```python
from build123d import *

# Parameters (mm, degrees)
BOSS_EXTRUDE2_DEPTH = 15
SKETCH3_W           = 40
SKETCH3_H           = 15
BOSS_EXTRUDE3_DEPTH = 10
BOSS_EXTRUDE4_START = -50
SKETCH4_R           = 5
BOSS_EXTRUDE4_DEPTH = 60
SKETCH5_W           = 20
SKETCH5_H           = 15
BOSS_EXTRUDE5_DEPTH = 10
BOSS_EXTRUDE6_START = -20
SKETCH6_R           = 5
BOSS_EXTRUDE6_DEPTH = 30
SKETCH7_W           = 20
SKETCH7_H           = 60
BOSS_EXTRUDE7_DEPTH = 60
SKETCH9_R           = 15
CUT_EXTRUDE1_DEPTH  = 5
SKETCH10_R          = 18
CUT_EXTRUDE2_DEPTH  = 5
FILLET1_R           = 30
FILLET2_R           = 5


with BuildPart() as part:
    # Sketch1 → Boss-Extrude2 (new body)
    with BuildSketch(Plane(origin=(0, 0, 0), x_dir=(1, 0, 0), z_dir=(0, 1, 0))):
        Polygon((0, 0), (300, 0), (300, -45), (180, -60), (20, -60), (20, -30), (0, -30), align=None)
    boss_extrude2 = extrude(amount=BOSS_EXTRUDE2_DEPTH)

    # Sketch3 → Boss-Extrude3 (add)
    with BuildSketch(Plane.XY.offset(60)):
        with Locations((160, 7.5)):
            Rectangle(SKETCH3_W, SKETCH3_H)
    boss_extrude3 = extrude(amount=BOSS_EXTRUDE3_DEPTH)

    # Sketch4 → Boss-Extrude4 (add)
    with BuildSketch(Plane(origin=(180, 0, 0), x_dir=(0, 0, -1), z_dir=(1, 0, 0)).offset(BOSS_EXTRUDE4_START)):
        with Locations((-70, 7.5)):
            Circle(SKETCH4_R)
    boss_extrude4 = extrude(amount=BOSS_EXTRUDE4_DEPTH)

    # Sketch5 → Boss-Extrude5 (add)
    with BuildSketch(Plane(origin=(300, 0, 0), x_dir=(0, 0, -1), z_dir=(1, 0, 0))):
        with Locations((-10, 7.5)):
            Rectangle(SKETCH5_W, SKETCH5_H)
    boss_extrude5 = extrude(amount=BOSS_EXTRUDE5_DEPTH)

    # Sketch6 → Boss-Extrude6 (add)
    with BuildSketch(Plane.XY.offset(20).offset(BOSS_EXTRUDE6_START)):
        with Locations((310, 7.5)):
            Circle(SKETCH6_R)
    boss_extrude6 = extrude(amount=BOSS_EXTRUDE6_DEPTH)

    # Mirror1: Boss-Extrude2, Boss-Extrude3, Boss-Extrude4, Boss-Extrude5, Boss-Extrude6 across plane
    add(boss_extrude2.mirror(Plane(origin=(0, 15, 0), x_dir=(1, 0, 0), z_dir=(0, 0, 1))))
    add(boss_extrude3.mirror(Plane(origin=(0, 15, 0), x_dir=(1, 0, 0), z_dir=(0, 0, 1))))
    add(boss_extrude4.mirror(Plane(origin=(0, 15, 0), x_dir=(1, 0, 0), z_dir=(0, 0, 1))))
    add(boss_extrude5.mirror(Plane(origin=(0, 15, 0), x_dir=(1, 0, 0), z_dir=(0, 0, 1))))
    add(boss_extrude6.mirror(Plane(origin=(0, 15, 0), x_dir=(1, 0, 0), z_dir=(0, 0, 1))))

    # Sketch7 → Boss-Extrude7 (add)
    with BuildSketch(Plane(origin=(0, 0, 0), x_dir=(1, 0, 0), z_dir=(0, 1, 0))):
        with Locations((10, 0)):
            Rectangle(SKETCH7_W, SKETCH7_H)
    extrude(amount=BOSS_EXTRUDE7_DEPTH)

    # Sketch9 → Cut-Extrude1 (cut)
    with BuildSketch(Plane.ZY):
        with Locations((0, 35)):
            Circle(SKETCH9_R)
    extrude(amount=-CUT_EXTRUDE1_DEPTH, mode=Mode.SUBTRACT)

    # Sketch10 → Cut-Extrude2 (cut)
    with BuildSketch(Plane.ZY.offset(-5)):
        with Locations((0, 35)):
            Circle(SKETCH10_R)
    extrude(amount=-CUT_EXTRUDE2_DEPTH, mode=Mode.SUBTRACT)

    # Fillet1
    fillet1_edges = [part.edges().sort_by_distance(p)[0] for p in [
        (10, 60, -30),
        (10, 60, 30),
    ]]
    fillet(fillet1_edges, radius=FILLET1_R - 0.0001)  # a hair under: the kernel refuses the full size

    # Fillet2
    fillet2_edges = [part.edges().sort_by_distance(p)[0] for p in [
        (20, 22.50005, -30),
        (20, 51.213232725, -21.213232725),
        (20, 22.50005, 30),
        (240, 15, -52.5),
        (300, 15, -32.5),
        (305, 15, -20),
        (305, 15, 20),
        (300, 15, 32.5),
        (240, 15, 52.5),
        (80, 15, -60),
        (80, 15, 60),
        (20, 51.213232725, 21.213232725),
    ]]
    fillet(fillet2_edges, radius=FILLET2_R)


solid = part.part
```
Model file for the job. Use its own axes, mm. A direction names the side the tool comes from. Round coordinates to 2 decimals unless told otherwise and drop trailing zeros. Write each loop counter-clockwise with the first axis right and the second up, starting at its lowest first coordinate (ties: lowest second). Pieces come first, ordered by that corner, then holes. Notation, with made-up numbers: M 78,65 L 132,65 A20 ccw 132,77 Z; hole C -9,52 d2. An arc over 180 degrees is marked long. Put each result on its own line as item: value.
Item 1: Cut at C-C (x = 31). List the corners of the cut face in (y, z).
Responses:
outline: M 0,-60 L 10,-60 A5 ccw 15,-55 L 15,55 A5 ccw 10,60 L 0,60 Z
Item 2: Cut at B-B (z = 35). List the corners of the cut face in (x, y).
Responses:
outline: M 20,0 L 300,0 L 300,10 A5 ccw 295,15 L 20,15 Z
Item 3: Mould opens along X. For faces 5 (the cylindrical face through (314.77, 9, -0.42)), 6 (the flat face through (0, 16, 0)), 7 (the flat face through (310, 8, -30)) say: +X half, -X half, draft (parallel to the pull), parting line (faces both ways), or undercut.
Responses:
face 5: undercut
face 6: -X half
face 7: draft
Item 4: Flat gauge pins, fed straight in: P1, Ø0.8, axis at x = 158, y = 1.5, coming from the +Z side; P2, Ø20, axis at y = 33.5, z = 4, coming from the +X side; P3, Ø5, axis at x = 308, y = 7, coming from the -Z side. Where does each tip first touch, or does it go through?
Responses:
P1: z = 70
P2: x = 20
P3: z = -30
Item 5: Tool access for faces 1 (the flat face through (190, 8, 70)), 2 (the flat face through (190, 8, -70)), 3 (the cylindrical face through (7.465, 52.847, -2.343)), 4 (the flat face through (20, 7, 45)): list every direction of +Z, -Z, +X, -X, +Y, -Y with a clear straight run to the whole face (end or side of a thin tool).
Responses:
face 1: +Z, +X, +Y, -Y
face 2: -Z, +X, +Y, -Y
face 3: none
face 4: +Z, -X, +Y, -Y
Item 6: Probe L1, parallel to Y at x = 1.9, z = 0; L2, parallel to Y at x = 6.3, z = 0; L3, parallel to Y at x = 48.5, z = 38. List the from-to ranges inside material, lowest first. Write a range as from..to.
Responses:
L1: 0..20, 50..60
L2: 0..17, 53..60
L3: 0..15
Item 7: Cut at A-A (x = 177). List the corners of the cut face in (y, z).
Responses:
outline: M 0,-70 L 2.5,-70 A5 ccw 12.5,-70 L 15,-70 L 15,70 L 12.5,70 A5 ccw 2.5,70 L 0,70 Z
